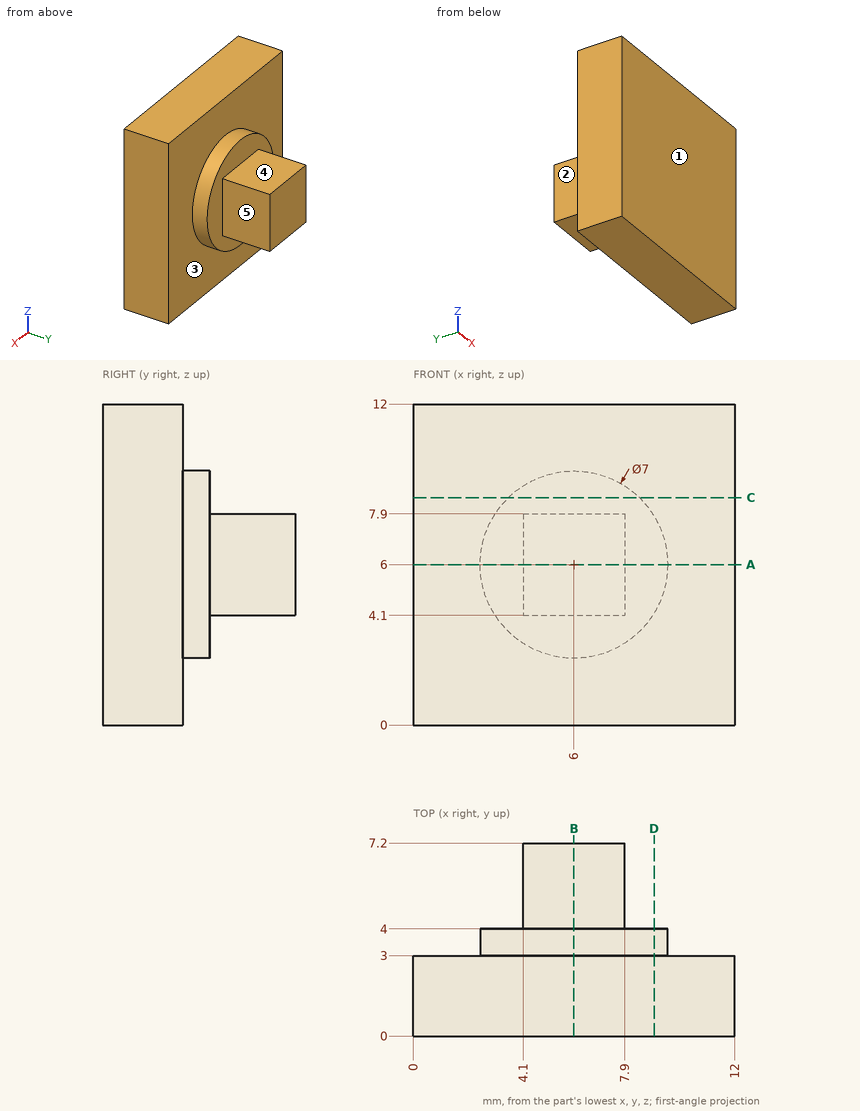
Input: dimensioned drawing with shaded views. Units: mm. Origin: part minimum x, y, z. A direction names the side the tool comes from. Round coordinates to 2 decimals unless told otherwise and drop trailing zeros. Loops run counter-clockwise (first coordinate to the right, second up) from the corner with the lowest first, then second, coordinate; pieces in that order, holes last. Notation, with made-up numbers: M 84.25,16 L 139.25,16 A25 cw 139.25,41 Z; hole C -29,-28 d8. An arc over 180 degrees is marked long. Return JSON: item names as keys, results as strings. Group by question number.
1. Pin query (flat end, axial travel): pin 1 (4 mm diameter, centred on x = 2, z = 2, fed in from +Y); pin 2 (1 mm diameter, centred on x = 10.5, y = 5, fed in from -Z); pin 3 (4 mm diameter, centred on x = 9.5, y = 6, fed in from +Z); pin 4 (3.5 mm diameter, centred on y = 6, z = 6.5, fed in from -X). Return the tip coordinate at first contact, or that it passes through.
2. Section query A-A on z = 6. Output: boundary loops of the cut face in (x, y).
3. Material intervals for line 1 along Y through (x, z) = (1.75, 11.75); line 2 along Y through (x, z) = (8, 4); line 3 along Z through (x, y) = (7, 4.75), sorted ascending. Write a range as from..to.
4. Section query C-C on z = 8.5. Output: boundary loops of the cut face in (x, y), and give its area (3 significant figures).
5. Reachability of the marked faces 1, 2, 3, 4 and 5 from +Z, -Z, +X, -X, +Y, -Y: full face, straight path, thin tool, end or side. Return the list, or none.
6. Section query D-D on x = 9. Output: boundary loops of the cut face in (y, z).
7. Section query B-B on x = 6. Output: boundary loops of the cut face in (y, z).
Checks:
{
 "1": {"pin 1": "stops at y = 3", "pin 2": "passes through", "pin 3": "stops at z = 7.9", "pin 4": "stops at x = 4.1"},
 "2": {"outline": "M 0,0 L 12,0 L 12,3 L 9.5,3 L 9.5,4 L 7.9,4 L 7.9,7.2 L 4.1,7.2 L 4.1,4 L 2.5,4 L 2.5,3 L 0,3 Z"},
 "3": {"line 1": "y = 0..3", "line 2": "y = 0..4", "line 3": "z = 4.1..7.9"},
 "4": {"outline": "M 0,0 L 12,0 L 12,3 L 8.45,3 L 8.45,4 L 3.55,4 L 3.55,3 L 0,3 Z", "area": "40.9 mm²"},
 "5": {"face 1": "+Z, -Z, +X, -X, -Y", "face 2": "+Z, -Z, -X, +Y", "face 3": "+Y", "face 4": "+Z, +X, -X, +Y", "face 5": "+Z, -Z, +X, +Y"},
 "6": {"outline": "M 0,0 L 3,0 L 3,4.2 L 4,4.2 L 4,7.8 L 3,7.8 L 3,12 L 0,12 Z"},
 "7": {"outline": "M 0,0 L 3,0 L 3,2.5 L 4,2.5 L 4,4.1 L 7.2,4.1 L 7.2,7.9 L 4,7.9 L 4,9.5 L 3,9.5 L 3,12 L 0,12 Z"}
}
